Build history of the part. All positions in model axes, mm. A direction names the side the tool comes from. Coordinates: 2 decimals unless noted, no trailing zeros. Write each loop counter-clockwise with the first axis right and the second up, starting at its lowest first coordinate (ties: lowest second). Pieces come first, ordered by that corner, then holes.
```python
from build123d import *

# Parameters (mm, degrees)
SKETCH1_R                       = 4.5
BOSS_EXTRUDE1_DEPTH             = 6.35
BOSS_EXTRUDE1_2_DEPTH           = 6.35
BOSS_EXTRUDE2_DEPTH             = 3.175
BOSS_EXTRUDE3_DEPTH             = 12.7
BOSS_EXTRUDE3_DIRECTION_2_REACH = 85.603
FILLET1_R                       = 5.08
FILLET2_R                       = 10.16
F_6_CLEARANCE_HOLE1_D           = 3.7973
F_6_CLEARANCE_HOLE1_DEPTH       = 6.35
FILLET5_START                   = -12.7
FILLET5_DEPTH                   = 17.2
CUT_EXTRUDE1_START              = -56.211523666
CUT_EXTRUDE1_DEPTH              = 56.211523666
BOSS_EXTRUDE5_REACH             = 132.89
BOSS_EXTRUDE5_END_RADIUS        = 5.715
SKETCH8_W                       = 9.525
SKETCH8_H                       = 3.175
FILLET6_R                       = 5.08
FILLET7_R                       = 2.54


with BuildPart() as part:
    # Sketch1 → Boss-Extrude1 (new body)
    with BuildSketch(Plane(origin=(0, 0, 0), x_dir=(1, 0, 0), z_dir=(0, 1, 0))):
        with Locations(Location((78.74, 0, 0), (0, 0, 270))):
            Circle(SKETCH1_R)
    extrude(amount=BOSS_EXTRUDE1_DEPTH)



with BuildPart() as body_2:
    # Sketch1 → Boss-Extrude1 2 (new body)
    with BuildSketch(Plane(origin=(0, 0, 0), x_dir=(1, 0, 0), z_dir=(0, 1, 0))):
        with Locations(Location((-78.74, 0, 0), (0, 0, 90))):
            Circle(SKETCH1_R)
    extrude(amount=BOSS_EXTRUDE1_2_DEPTH)


with BuildPart() as part_1:
    add(part.part)

    add(body_2.part)  # Boss-Extrude2 merges body 2
    # Sketch2 → Boss-Extrude2 (add)
    with BuildSketch(Plane(origin=(0, 0, 0), x_dir=(1, 0, 0), z_dir=(0, 1, 0))):
        with BuildLine():
            Line((78.74, 4.5), (-78.74, 4.5))
            ThreePointArc((-78.74, 4.5), (-75.558019485, 3.181980515), (-74.24, 0))
            ThreePointArc((-74.24, 0), (-75.558019485, -3.181980515), (-78.74, -4.5))
            Line((-78.74, -4.5), (78.74, -4.5))
            ThreePointArc((78.74, -4.5), (74.24, 0), (78.74, 4.5))
        make_face()
    extrude(amount=BOSS_EXTRUDE2_DEPTH)

    # Sketch3 → Boss-Extrude3 (add)
    with BuildSketch(Plane.XY):
        with BuildLine():
            Line((-78.74, 0), (-78.74, 3.175))
            Line((-78.74, 3.175), (-90.114089339, 3.175))
            ThreePointArc((-90.114089339, 3.175), (-88.335814095, 20.989027697), (-83.071170469, 38.1))
            Line((-83.071170469, 38.1), (16.51, 38.1))
            Line((16.51, 38.1), (16.51, 44.45))
            Line((16.51, 44.45), (-80.105931514, 44.45))
            ThreePointArc((-80.105931514, 44.45), (-75.082403553, 53.007088382), (-69.148535375, 60.96))
            Line((-69.148535375, 60.96), (16.51, 60.96))
            Line((16.51, 60.96), (16.51, 64.77))
            Line((16.51, 64.77), (-71.560865702, 64.77))
            ThreePointArc((-71.560865702, 64.77), (-90.064324673, 34.70630809), (-96.52, 0))
            Line((-96.52, 0), (-78.74, 0))
        make_face()
    extrude(amount=-BOSS_EXTRUDE3_DEPTH)

    # Boss-Extrude3 direction 2: up to this face of the body (flat: up to its plane)
    boss_extrude3_direction_2_end = Plane(part_1.part.faces().sort_by_distance((0, 1.5875, 4.5))[0])
    # Sketch3 → Boss-Extrude3 direction 2 (add, up to the picked face)
    with BuildSketch(Plane.XY, mode=Mode.PRIVATE) as boss_extrude3_direction_2_sk1:
        with BuildLine():
            Line((-78.74, 0), (-78.74, 3.175))
            Line((-78.74, 3.175), (-90.114089339, 3.175))
            ThreePointArc((-90.114089339, 3.175), (-88.335814095, 20.989027697), (-83.071170469, 38.1))
            Line((-83.071170469, 38.1), (16.51, 38.1))
            Line((16.51, 38.1), (16.51, 44.45))
            Line((16.51, 44.45), (-80.105931514, 44.45))
            ThreePointArc((-80.105931514, 44.45), (-75.082403553, 53.007088382), (-69.148535375, 60.96))
            Line((-69.148535375, 60.96), (16.51, 60.96))
            Line((16.51, 60.96), (16.51, 64.77))
            Line((16.51, 64.77), (-71.560865702, 64.77))
            ThreePointArc((-71.560865702, 64.77), (-90.064324673, 34.70630809), (-96.52, 0))
            Line((-96.52, 0), (-78.74, 0))
        make_face()
    boss_extrude3_direction_2_tool1 = split(extrude(boss_extrude3_direction_2_sk1.sketch, amount=BOSS_EXTRUDE3_DIRECTION_2_REACH, mode=Mode.PRIVATE), bisect_by=boss_extrude3_direction_2_end, keep=Keep.BOTH, mode=Mode.PRIVATE)
    add(boss_extrude3_direction_2_tool1.solids().sort_by(Axis((-47.115631, 42.638129, 0), (0, 0, 1)))[0])

    # Fillet1
    fillet1_edges = [part_1.edges().sort_by_distance(p)[0] for p in [
        (-69.148535375, 60.96, -4.1),
        (-90.114089339, 3.175, -4.1),
    ]]
    fillet(fillet1_edges, radius=FILLET1_R)

    # Fillet2
    # the kernel refuses this fillet: 10.16 mm, written as the material it adds along each edge
    with BuildSketch(Plane(origin=(-78.74, 0, -4.5), x_dir=(1, 0, 0), z_dir=(0, 1, 0))) as fillet2_piece_1:
        with BuildLine():
            CenterArc((9.969152421, 10.16), FILLET2_R, 191.12285511, 78.87714489)
            Line((0, 8.2), (0, 0))
            Line((0, 0), (9.969152421, 0))
        make_face()
    extrude(amount=3.175)
    # the kernel refuses this fillet: 10.16 mm, written as the material it takes off along each edge
    with BuildSketch(Plane(origin=(-71.560865702, 64.77, 16.814827808), x_dir=(1, 0, 0), z_dir=(0, 0, -1))) as fillet2_2_piece_1:
        with BuildLine():
            CenterArc((4.659464371, 10.16), FILLET2_R, 219.223932399, 50.776067601)
            ThreePointArc((-3.211288726, 3.735294118), (-1.629477245, 1.847157571), (0, 0))
            Line((0, 0), (4.659464371, 0))
        make_face()
    extrude(amount=41.829655616, mode=Mode.SUBTRACT)

    # #6 Clearance Hole1
    with Locations(Plane(origin=(-78.74, 6.35, 0), x_dir=(0, 0, 1), z_dir=(0, 1, 0))):
        with Locations((0, 0), (0, 157.48)):
            Hole(F_6_CLEARANCE_HOLE1_D / 2, depth=F_6_CLEARANCE_HOLE1_DEPTH)

    # Fillet5: read off the stored shape, not the designer's step
    # Fillet5 outline → Fillet5 (add)
    with BuildSketch(Plane.XY.offset(FILLET5_START)):
        with BuildLine():
            add(Edge.make_bspline(
                [(-57.486261954, 38.1), (-84.476947832, 38.1), (-89.953142639, 8.558476434)],
                knots=[0, 0, 0, 1, 1, 1], degree=2, weights=[1, 0.768852264, 1]))
            Line((-57.486261954, 38.1), (-83.071170469, 38.1))
            ThreePointArc((-83.071170469, 38.1), (-87.76402471, 23.620872526), (-89.953142639, 8.558476434))
        make_face()
    extrude(amount=FILLET5_DEPTH)

    # Cut-Extrude1: read off the stored shape, not the designer's step
    # Cut-Extrude1 outline → Cut-Extrude1 (cut)
    with BuildSketch(Plane(origin=(0, 64.77, 0), x_dir=(1, 0, 0), z_dir=(0, 1, 0)).offset(CUT_EXTRUDE1_START)):
        with BuildLine():
            Line((-82.262956855, -4.5), (-75.217043145, -4.5))
            ThreePointArc((-75.217043145, -4.5), (-78.74, 5.715), (-82.262956855, -4.5))
        make_face()
    extrude(amount=CUT_EXTRUDE1_DEPTH, mode=Mode.SUBTRACT)

    # Boss-Extrude5: up to this cylinder (the profile starts outside it)
    boss_extrude5_end = Plane(origin=(-78.74, 46.0375, 0), z_dir=(0, 1, 0)) * Cylinder(BOSS_EXTRUDE5_END_RADIUS, 278.21, mode=Mode.PRIVATE)
    # Sketch8 → Boss-Extrude5 (add, up to the surface)
    with BuildSketch(Plane(origin=(16.51, 0, 0), x_dir=(0, 0, -1), z_dir=(1, 0, 0)), mode=Mode.PRIVATE) as boss_extrude5_sk1:
        with Locations((0.2625, 46.0375)):
            Rectangle(SKETCH8_W, SKETCH8_H)
    boss_extrude5_tool1 = extrude(boss_extrude5_sk1.sketch, amount=-BOSS_EXTRUDE5_REACH, mode=Mode.PRIVATE) - boss_extrude5_end
    add(boss_extrude5_tool1.solids().sort_by_distance((16.51, 46.0375, -0.2625))[0])

    # Fillet6
    # the kernel refuses this fillet: 5.08 mm, written as the material it adds along each edge
    with BuildSketch(Plane(origin=(16.51, 44.45, -5.025), x_dir=(0, 1, 0), z_dir=(-1, 0, 0))) as fillet6_piece_1_section:
        with BuildLine():
            CenterArc((5.08, 4.709286039), FILLET6_R, 180, 67.975687163)
            Line((0, 4.709286039), (0, 0))
            Line((0, 0), (3.175, 0))
        make_face()
    fillet6_piece_1 = extrude(amount=104.300973375, mode=Mode.PRIVATE)
    fillet6_piece_1 = fillet6_piece_1 - Plane(origin=(-78.74, 44.45, 0), x_dir=(1, 0, 0), z_dir=(0, 1, 0)) * Cylinder(5.715, 228, mode=Mode.PRIVATE)
    fillet6_piece_1 = fillet6_piece_1 & Plane(origin=(0, 0, -5.025), x_dir=(-0.7414097151042524, 0.671052631578948, 0), z_dir=(0, 0, 1)) * Cylinder(96.52, 228, mode=Mode.PRIVATE)
    add(fillet6_piece_1)

    # Fillet7
    fillet7_edges = [part_1.edges().sort_by_distance(p)[0] for p in [
        (16.51, 47.625, -0.2625),
        (16.51, 60.96, -4.1),
    ]]
    fillet(fillet7_edges, radius=FILLET7_R)


solid = part_1.part
```
1. Mould opens along Y. For faces 4 (the face through (-21, 38.1, -4)), 5 (the face through (80.622, 3.131, 0.247)), 6 (the face through (-71.314, 63.762, -3.98)), 7 (the face through (-30, 47.625, 0)) say: +Y half, -Y half, draft (parallel to the pull), parting line (faces both ways), or undercut.
Computed values:
face 4: undercut
face 5: draft
face 6: +Y half
face 7: undercut
2. Flat gauge pins, fed straight in: pin 1 (1 mm diameter, centred on y = 64, z = -0.5, fed in from +X); pin 2 (7 mm diameter, centred on x = 81, z = -1.5, fed in from +Y); pin 3 (3.5 mm diameter, centred on x = 33, y = 1.5, fed in from -Z); pin 4 (2.5 mm diameter, centred on x = -78.74, z = 0, fed in from +Y). Where does each tip first touch, or does it go through?
Computed values:
pin 1: stops at x = 16.51
pin 2: stops at y = 6.35
pin 3: stops at z = -4.5
pin 4: passes through
3. Probe line 1 along Y through (x, z) = (-51, 1.5) (3 decimals); line 2 along Y through (x, z) = (-15, -9.25); line 3 along Y through (x, z) = (-23, -5) (3 decimals). List the from-to ranges inside material, lowest first.
Computed values:
line 1: y = 0 to 3.175, 38.1 to 47.625, 60.96 to 64.77
line 2: y = 38.1 to 44.47, 60.96 to 64.77
line 3: y = 38.1 to 47.625, 60.96 to 64.77
4. 3-axis set-ups, long thin cutter, end or side, ignore diameter. For faces 1 (the face through (83.2, 3.8, -0.6)), 2 (the face through (-31, 44.45, -11)), 3 (the face through (-75.3, 1.565, -6.876)): which of +Z, -Z, +X, -X, +Y, -Y reach the whole face in a straight line?
Computed values:
face 1: +Y
face 2: -Z, +X
face 3: -Z, +X, -Y
5. Saw through at B-B on x = 37.5. List the corners of the cut face in (y, z) (3 decimals), plus the area to 3 significant figures.
Computed values:
outline: (0, -4.5) - (3.175, -4.5) - (3.175, 4.5) - (0, 4.5) - close
area: 28.6 mm2
6. Saw through at C-C on z = 0. State how many separate pieces and enclosed holes the cut face has, plus the area to 3 significant figures.
Computed values:
separate pieces: 5
enclosed holes: 0
area: 2,070 mm2
7. Saw through at A-A on x = -15.5. List the corners of the cut face in (y, z) (3 decimals).
Computed values:
outline: (0, -4.5) - (3.175, -4.5) - (3.175, 4.5) - (0, 4.5) - close; (38.1, -12.7) - (44.45, -12.7) - (44.45, -9.734) arc R5.08 cw to (47.625, -5.025) - (47.625, 4.5) - (38.1, 4.5) - close; (60.96, -12.7) - (64.77, -12.7) - (64.77, 4.5) - (60.96, 4.5) - close
